```python
from build123d import *

# Parameters (mm, degrees)
F0_W     = 31.6738
F0_H     = 7.6962
F1_DEPTH = 9.4488
F2_R     = 2.4003
F3_DEPTH = 1.7526
F4_W     = 29.3116
F4_H     = 6.1722
F5_DEPTH = 8.128
F6_R     = 1.4605
F7_DEPTH = 8.128


with BuildPart() as f1:
    # F0 (on Top) → F1 (new body)
    with BuildSketch(Plane.XY):
        Rectangle(F0_W, F0_H)
    extrude(amount=F1_DEPTH)

    # F2 (on face) → F3 (join)
    with BuildSketch(Plane.XY.offset(9.4488)):
        with Locations((-12.0396, 0)):
            Circle(F2_R)
        with Locations((-3.7846, 0)):
            Circle(F2_R)
        with Locations((3.7846, 0)):
            Circle(F2_R)
        with Locations((12.0396, 0)):
            Circle(F2_R)
    extrude(amount=F3_DEPTH)

    # F4 (on face) → F5 (cut)
    with BuildSketch(Plane(origin=(0, 0, 0), x_dir=(1, 0, 0), z_dir=(0, 0, -1))):
        Rectangle(F4_W, F4_H)
    extrude(amount=-F5_DEPTH, mode=Mode.SUBTRACT)

    # F6 (on face) → F7 (join)
    with BuildSketch(Plane(origin=(0, 0, 8.128), x_dir=(1, 0, 0), z_dir=(0, 0, -1))):
        Circle(F6_R)
        with Locations((8.731115, 0)):
            Circle(F6_R)
        with Locations((-8.370964, 0)):
            Circle(F6_R)
    extrude(amount=F7_DEPTH)


solid = f1.part
```
Source: CAD feature listing. Evaluate the final solid. Frame: model axes, mm. A direction names the side the tool comes from. Coordinates: 2 decimals unless noted, no trailing zeros. Order: outer loops, then holes, each group sorted by start corner. A loop starts at its lowest first (then second) coordinate and runs counter-clockwise, first axis right, second up. Notation, with made-up numbers: M -6.75,76.25 L 36.25,76.25 A21 ccw 36.25,103.25 Z; hole C -13,81 d2. An arc over 180 degrees is marked long. Write each question's results on one line, items separated by ' | '. Start each with the question number.
1) Line query: line 1 (Y direction, x = 4, z = 2.5); line 2 (X direction, y = -3, z = 4); line 3 (Y direction, x = -9, z = 1.25). Output: solid intervals per line, ascending. Write a range as from..to.
2) Section query C-C (y = 2). Return the cut outline in (x, z).
3) Draft query along Y for faces 1 (the face through (-12, 0, 11.201)), 2 (the face through (10.124, -0.439, 4.121)), 3 (the face through (0, 3.848, 5)). Return one class per face: released by +Y, released by -Y, zero draft, split by the parting line, or undercut.
4) Section query B-B (x = 0). Return the cut outline in (y, z), plus the area to 3 significant figures.
5) Contact query for a flat-ended pin moving along its axis: pin 1 Ø3 at (x, y) = (3.5, 0) entering from -Z. Output: stop coordinate, or through.
6) Section query A-A (z = 2). Return the cut outline in (x, y), plus the area to 3 significant figures.
7) Access query for faces 4 (the face through (-8.688, 1.426, 4.121)), 5 (the face through (0, -3.848, 5)), 6 (the face through (0, 0, 9.449)). Directions: +Z, -Z, +X, -X, +Y, -Y. A direction counts if a zero-diameter tool reaches every point of the face in a straight line with its end or side. Return the directions, or none.
8) Section query D-D (x = -7.5). Return the cut outline in (y, z), plus the area to 3 significant figures.
Answers:
1) line 1: y = -3.85..-3.09, 3.09..3.85 | line 2: x = -15.84..-14.66, 14.66..15.84 | line 3: y = -3.85..-3.09, -1.32..1.32, 3.09..3.85
2) outline: M -15.84,0 L -14.66,0 L -14.66,8.13 L 14.66,8.13 L 14.66,0 L 15.84,0 L 15.84,9.45 L 13.37,9.45 L 13.37,11.2 L 10.71,11.2 L 10.71,9.45 L 5.11,9.45 L 5.11,11.2 L 2.46,11.2 L 2.46,9.45 L -2.46,9.45 L -2.46,11.2 L -5.11,11.2 L -5.11,9.45 L -10.71,9.45 L -10.71,11.2 L -13.37,11.2 L -13.37,9.45 L -15.84,9.45 Z
3) face 1: zero draft | face 2: undercut | face 3: released by +Y
4) outline: M -3.85,0 L -3.09,0 L -3.09,8.13 L -1.46,8.13 L -1.46,0 L 1.46,0 L 1.46,8.13 L 3.09,8.13 L 3.09,0 L 3.85,0 L 3.85,9.45 L -3.85,9.45 Z | area: 46.3 mm^2
5) pin 1: stops at z = 8.13
6) outline: M -15.84,-3.85 L 15.84,-3.85 L 15.84,3.85 L -15.84,3.85 Z; C -8.37,0 d2.92; C 0,0 d2.92; C 8.73,0 d2.92; hole M -14.66,-3.09 L 14.66,-3.09 L 14.66,3.09 L -14.66,3.09 Z | area: 83.0 mm^2
7) face 4: -Z | face 5: +Z, -Z, +X, -X, -Y | face 6: +Z
8) outline: M -3.85,0 L -3.09,0 L -3.09,8.13 L -1.17,8.13 L -1.17,0 L 1.17,0 L 1.17,8.13 L 3.09,8.13 L 3.09,0 L 3.85,0 L 3.85,9.45 L -3.85,9.45 Z | area: 41.6 mm^2
